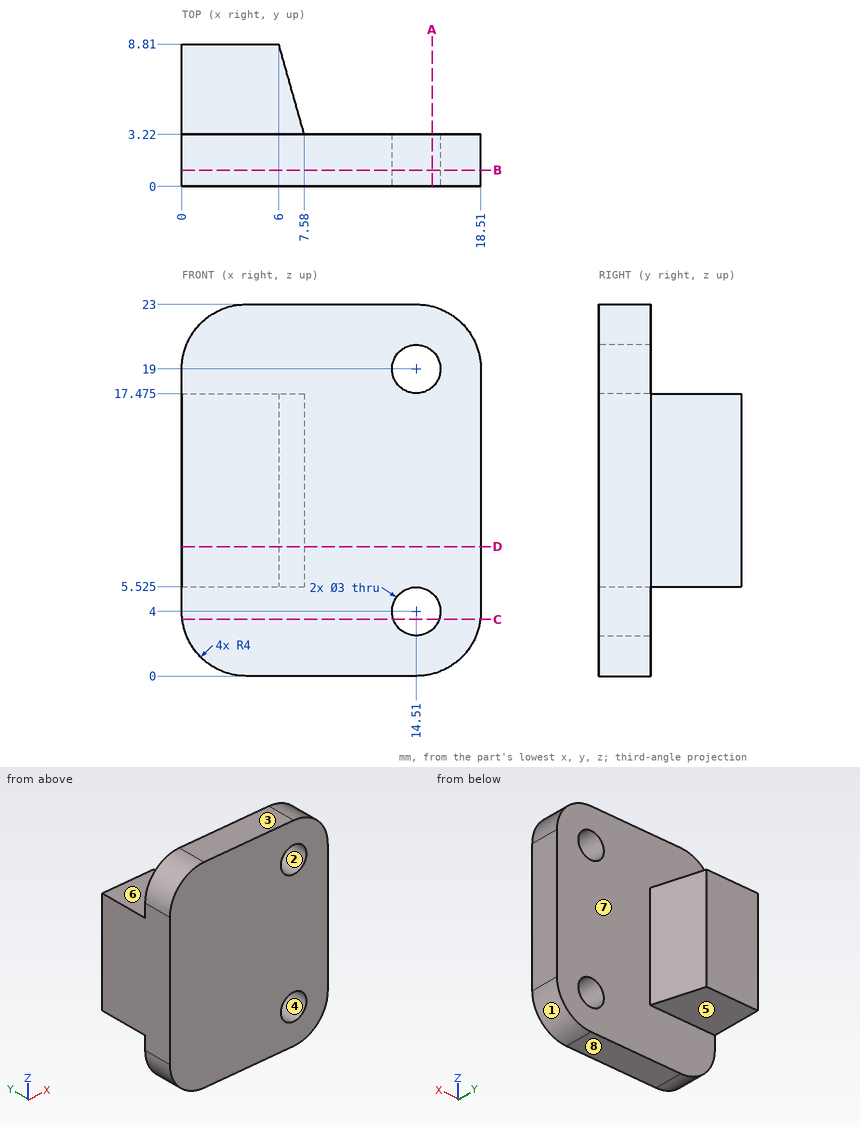
The figure shows three views and two pictorial views of one solid part (mm, origin at its lowest corner). Answer the questions. A direction names the side the tool comes from. Give positions to 0.01 mm unless a question says otherwise; leave off trailing zeros. Write each loop counter-clockwise with the first axis right and the second up, starting at its lowest first coordinate (ties: lowest second). Pieces come first, ordered by that corner, then holes. Notation, with made-up numbers: (88, 66) -> (95, 66) arc R17 ccw to (95, 92) -> close; hole circle Ø9 at (-19.75, 25.5). An arc over 180 degrees is marked (long way). Answer as a JSON object with one key per item and string values.
1) Section D-D on z = 8 is taken. Write down the section's boundary in (x, y), then the cut area to 3 significant figures.
Findings below:
{"outline": "(0, 0) -> (18.51, 0) -> (18.51, 3.22) -> (7.58, 3.22) -> (6, 8.81) -> (0, 8.81) -> close", "area": "97.6 mm^2"}
2) Flat-ended cylindrical pins translate along their axes: pin 1 Ø4.5 at (x, y) = (4, 5.5) entering from -Z (3 decimals); pin 2 Ø2.5 at (x, z) = (14.51, 19) entering from -Y; pin 3 Ø3 at (x, y) = (5, 5) entering from +Z (3 decimals). Find the tip coordinate at first contact, or state that the pin passes through.
Findings below:
{"pin 1": "stops at z = 5.525", "pin 2": "passes through", "pin 3": "stops at z = 17.475"}
3) Section C-C on z = 3.5 is taken. Write down the section's boundary in (x, y).
Findings below:
{"outline": "(0.03, 0) -> (13.1, 0) -> (13.1, 3.22) -> (0.03, 3.22) -> close; (15.92, 0) -> (18.48, 0) -> (18.48, 3.22) -> (15.92, 3.22) -> close"}
4) A tool of negligible diameter and unlimited length cuts with its end or side. For the marked faces 5, 6, 7 and 8, from which of +Z, -Z, +X, -X, +Y, -Y can it reach the whole face along a straight path? Write none if from no direction.
Findings below:
{"face 5": "-Z, +X, -X, +Y", "face 6": "+Z, +X, -X, +Y", "face 7": "+X, +Y", "face 8": "-Z, +X, -X, +Y, -Y"}
5) Section B-B on y = 1 is taken. Write down the section's boundary in (x, z), then the cut area to 3 significant figures.
Findings below:
{"outline": "(0, 4) arc R4 ccw to (4, 0) -> (14.51, 0) arc R4 ccw to (18.51, 4) -> (18.51, 19) arc R4 ccw to (14.51, 23) -> (4, 23) arc R4 ccw to (0, 19) -> close; hole circle Ø3 at (14.51, 4); hole circle Ø3 at (14.51, 19)", "area": "398 mm^2"}
6) For a pull along X with two mould halves and no side action, classify the marked faces 1, 2, 3 and 4 as pulls with the +X half, pulls with the -X half, needs draft (parallel to the pull), parting line crosses it, or undercut.
Findings below:
{"face 1": "pulls with the +X half", "face 2": "undercut", "face 3": "needs draft", "face 4": "undercut"}
7) Straight lines are drawn through the part: probe 1 along Z at (x, y) = (14.51, 0.75); probe 2 along X at (y, z) = (2, 19); probe 3 along Z at (x, y) = (15, 2.25). For each, find the intervals that lie inside material, in ascending order. Write a range as from..to.
Findings below:
{"probe 1": "z = 0..2.5, 5.5..17.5, 20.5..23", "probe 2": "x = 0..13.01, 16.01..18.51", "probe 3": "z = 0.03..2.58, 5.42..17.58, 20.42..22.97"}
8) Section A-A on x = 15.5 is taken. Write down the section's boundary in (y, z).
Findings below:
{"outline": "(0, 0.12) -> (3.22, 0.12) -> (3.22, 2.87) -> (0, 2.87) -> close; (0, 5.13) -> (3.22, 5.13) -> (3.22, 17.87) -> (0, 17.87) -> close; (0, 20.13) -> (3.22, 20.13) -> (3.22, 22.88) -> (0, 22.88) -> close"}
